Part model, mm, in its own coordinate system. A direction names the side the tool comes from. Round coordinates to 2 decimals unless told otherwise and drop trailing zeros. Loops run counter-clockwise (first coordinate to the right, second up) from the corner with the lowest first, then second, coordinate; pieces in that order, holes last. Notation, with made-up numbers: M 45.5,-16.5 L 73.5,-16.5 A17 cw 73.5,-5.5 Z; hole C -1,21.25 d3. An arc over 180 degrees is marked long. Answer as CSV lines item,"result". Start each with the question number.
Item 1: Drop flat-ended pins along their axis: pin 1 Ø7 at (x, z) = (0, 15) entering from -Y; pin 2 Ø1.5 at (x, y) = (-217.5, -83) entering from -Z. Give the stop position or say it passes through.
Item 2: Which spindle directions (+Z, -Z, +X, -X, +Y, -Y) get a long thin tool onto all of the face, cutting with end or side? Do faces 4 (the flat face through (-219, 15, 267)), 5 (the flat face through (-1, 218.5, 275)). Say none if no direction does.
Item 3: Band-saw the part on A-A (z = 66). Give the cut face in (x, y).
Item 4: Band-saw the part on C-C (y = -53). Give the cut face in (x, z).
Item 5: Band-saw the part on B-B (x = 43). Give the cut face in (y, z), and give its area (3 significant figures).
Item 6: Wall check: line 1 (Z direction, x = 0, y = -220); line 2 (X direction, y = 160, z = 270.5); line 3 (Y direction, x = -41.5, z = 275.5). Give the ranges that are in metal, low to high.
Item 7: Mould opens along Y. For faces 1 (the flat face through (15, 221.5, 267)), 2 (the flat face through (219, 15, 267)), 3 (the flat face through (216, -1, 275)) say: pulls with the +Y half, pulls with the -Y half, needs draft (parallel to the pull), parting line crosses it, or undercut.
```python
from build123d import *

# Parameters (mm, degrees)
F0_W          = 438
F0_H          = 443
F1_DEPTH      = 295
F2_T          = -3
F3_W          = 378
F3_H          = 265
F4_DEPTH      = 221.501
F4_DEPTH_BACK = 221.501
F5_W          = 383
F5_H          = 265
F6_DEPTH      = 219.001
F6_DEPTH_BACK = 219.001
F7_W          = 378
F7_H          = 383
F8_DEPTH      = 295.001
F9_W          = 378
F9_H          = 30
F9_R          = 4
F10_DEPTH     = 3
F11_R         = 4
F12_DEPTH     = 438.001


with BuildPart() as f1:
    # F0 (on Top) → F1 (new body)
    with BuildSketch(Plane.XY):
        Rectangle(F0_W, F0_H)
    extrude(amount=F1_DEPTH)

    # F2
    f2_openings = [f1.faces().sort_by_distance(p)[0] for p in [
        (0, 0, 0),
    ]]
    offset(amount=F2_T, openings=f2_openings)

    # F3 (on Front) → F4 (cut, two sides)
    with BuildSketch(Plane.XZ) as f4_sk:
        with Locations((0, 132.5)):
            Rectangle(F3_W, F3_H)
    extrude(amount=-F4_DEPTH, mode=Mode.SUBTRACT)
    extrude(f4_sk.sketch, amount=F4_DEPTH_BACK, mode=Mode.SUBTRACT)

    # F5 (on Right) → F6 (cut, two sides)
    with BuildSketch(Plane.YZ) as f6_sk:
        with Locations((0, 132.5)):
            Rectangle(F5_W, F5_H)
    extrude(amount=-F6_DEPTH, mode=Mode.SUBTRACT)
    extrude(f6_sk.sketch, amount=F6_DEPTH_BACK, mode=Mode.SUBTRACT)

    # F7 (on face) → F8 (cut, through all)
    with BuildSketch(Plane.XY.offset(295)):
        Rectangle(F7_W, F7_H)
    extrude(amount=-F8_DEPTH, mode=Mode.SUBTRACT)

    # F9 (on face) → F10 (join, through all)
    with BuildSketch(Plane.XZ.offset(221.5)):
        with Locations((0, 15)):
            Rectangle(F9_W, F9_H)
        with Locations((0, 15)):
            Circle(F9_R, mode=Mode.SUBTRACT)
    extrude(amount=-F10_DEPTH)

    # F11 (on face) → F12 (cut, through all)
    with BuildSketch(Plane.YZ.offset(219)):
        with Locations((206.5, 19)):
            Circle(F11_R)
    extrude(amount=-F12_DEPTH, mode=Mode.SUBTRACT)


solid = f1.part
```
Answer block:
1,pin 1,"passes through"
1,pin 2,"stops at z = 265"
2,face 4,"+Z, -Z, -X, +Y, -Y"
2,face 5,"-Z"
3,outline,"M -219,-221.5 L -189,-221.5 L -189,-218.5 L -216,-218.5 L -216,-191.5 L -219,-191.5 Z; M -219,191.5 L -216,191.5 L -216,218.5 L -189,218.5 L -189,221.5 L -219,221.5 Z; M 189,-221.5 L 219,-221.5 L 219,-191.5 L 216,-191.5 L 216,-218.5 L 189,-218.5 Z; M 189,218.5 L 216,218.5 L 216,191.5 L 219,191.5 L 219,221.5 L 189,221.5 Z"
4,outline,"M -219,265 L -216,265 L -216,292 L -189,292 L -189,295 L -219,295 Z; M 189,292 L 216,292 L 216,265 L 219,265 L 219,295 L 189,295 Z"
5,outline,"M -221.5,0 L -218.5,0 L -218.5,30 L -221.5,30 Z; M -221.5,265 L -218.5,265 L -218.5,292 L -191.5,292 L -191.5,295 L -221.5,295 Z; M 191.5,292 L 218.5,292 L 218.5,265 L 221.5,265 L 221.5,295 L 191.5,295 Z"
5,area,"432 mm^2"
6,line 1,"z = 0 to 11, 19 to 30, 265 to 295"
6,line 2,"x = -219 to -216, 216 to 219"
6,line 3,"y = -221.5 to -218.5, 218.5 to 221.5"
7,face 1,"pulls with the +Y half"
7,face 2,"needs draft"
7,face 3,"undercut"
